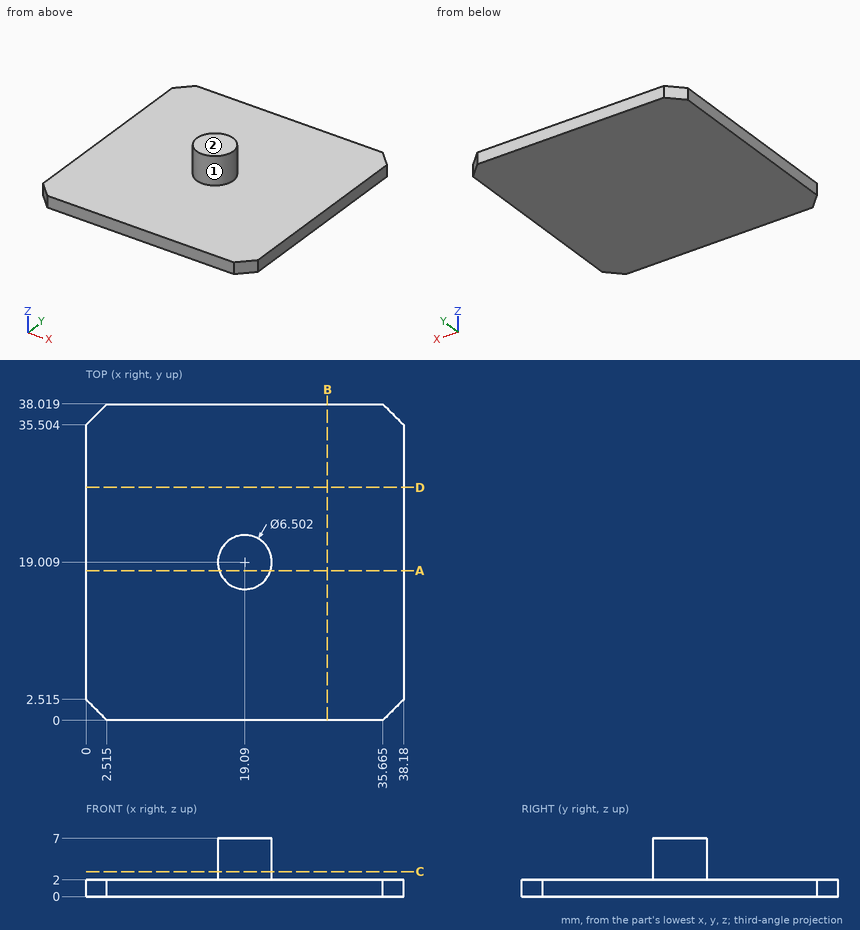
Answer from the drawing. Dimensions are ordinates in mm from the lowest x, y and z of the part. A direction names the side the tool comes from. Give positions to 0.01 mm unless a question says otherwise; leave off trailing zeros. Loops run counter-clockwise (first coordinate to the right, second up) from the corner with the lowest first, then second, coordinate; pieces in that order, holes last. Notation, with made-up numbers: (-22, 48.5) -> (34, 48.5) arc R12 cw to (34, 56.5) -> close; hole circle Ø10 at (-17, 85.25). An arc over 180 degrees is marked (long way). Use a Markdown table: item, result.
Q1. Section D-D, the plane y = 28 is taken. Determine the outline of the cut face in (x, z).
Solved:
| item | result |
|---|---|
| outline | (0, 0) -> (38.18, 0) -> (38.18, 2) -> (0, 2) -> close |
Q2. This flat-tipped pin is pushed along its axis until it touches: pin 1 (3 mm diameter, centred on x = 24, y = 18, fed in from +Z). Where does it stop, or does it pass through?
Solved:
| item | result |
|---|---|
| pin 1 | stops at z = 2 |
Q3. A tool of negligible diameter and unlimited length cuts with its end or side. For the marked faces 1 and 2, from which of +Z, -Z, +X, -X, +Y, -Y can it reach the whole face along a straight path? Write none if from no direction.
Solved:
| item | result |
|---|---|
| face 1 | +Z |
| face 2 | +Z, +X, -X, +Y, -Y |
Q4. Section A-A, the plane y = 18 is taken. Determine the outline of the cut face in (x, z).
Solved:
| item | result |
|---|---|
| outline | (0, 0) -> (38.18, 0) -> (38.18, 2) -> (22.18, 2) -> (22.18, 7) -> (16, 7) -> (16, 2) -> (0, 2) -> close |
Q5. Find the intervals of material crossed by line 1 along Z through (x, y) = (24, 19.5); line 2 along X through (y, z) = (17.5, 3.75); line 3 along Y through (x, z) = (22, 3.5) (1 decimal), in increasing order.
Solved:
| item | result |
|---|---|
| line 1 | z = 0 to 2 |
| line 2 | x = 16.21 to 21.97 |
| line 3 | y = 17.6 to 20.5 |
Q6. Section B-B, the plane x = 29 is taken. Determine the outline of the cut face in (y, z).
Solved:
| item | result |
|---|---|
| outline | (0, 0) -> (38.02, 0) -> (38.02, 2) -> (0, 2) -> close |
Q7. Section C-C, the plane z = 3 is taken. Determine the outline of the cut face in (x, y).
Solved:
| item | result |
|---|---|
| outline | circle Ø6.5 at (19.09, 19.01) |
